from build123d import *

# Parameters (mm, degrees)
SKIZZE2_W                       = 28
SKIZZE2_H                       = 4
AUFSATZ_LINEAR_AUSTRAGEN2_DEPTH = 17.9
SKIZZE4_W                       = 35.8
SKIZZE4_H                       = 28
AUFSATZ_LINEAR_AUSTRAGEN3_DEPTH = 5
SKIZZE7_W                       = 8.2
SKIZZE7_H                       = 3
SCHNITT_LINEAR_AUSTRAGEN4_DEPTH = 1.5
SKIZZE5_W                       = 33.2
SKIZZE5_H                       = 18.5
SCHNITT_LINEAR_AUSTRAGEN2_DEPTH = 4.3
SKIZZE8_W                       = 34.6
SKIZZE8_H                       = 28
SCHNITT_LINEAR_AUSTRAGEN5_DEPTH = 3.5
AUFSATZ_LINEAR_AUSTRAGEN4_DEPTH = 1.5
SKIZZE9_W                       = 33.2
SKIZZE9_H                       = 3
SCHNITT_LINEAR_AUSTRAGEN6_DEPTH = 1.5
SKIZZE11_W                      = 28
SKIZZE11_H                      = 4.8
AUFSATZ_LINEAR_AUSTRAGEN5_DEPTH = 1.2
SKIZZE12_W                      = 28
SKIZZE12_H                      = 4.75
AUFSATZ_LINEAR_AUSTRAGEN6_DEPTH = 3.65
SKIZZE13_R                      = 1.2
AUFSATZ_LINEAR_AUSTRAGEN7_DEPTH = 2.5
LINEARES_MUSTER1_COUNT          = 2
LINEARES_MUSTER1_PITCH          = 15.2
LINEARES_MUSTER1_COUNT_DIR2     = 2
LINEARES_MUSTER1_PITCH_DIR2     = 21.6
SCHNITT_LINEAR_AUSTRAGEN7_DEPTH = 14.8
VERRUNDUNG1_R                   = 0.2
SKIZZE20_W                      = 27.6
SKIZZE20_H                      = 4.65
AUFSATZ_LINEAR_AUSTRAGEN8_DEPTH = 1.3
VERRUNDUNG2_R                   = 1.5
SCHNITT_LINEAR_AUSTRAGEN8_DEPTH = 1


with BuildPart() as part:
    # Skizze2 → Aufsatz-Linear austragen2 (new body, symmetric)
    with BuildSketch(Plane(origin=(0, 0, 0), x_dir=(0, 0, -1), z_dir=(1, 0, 0))):
        with Locations((0, -2)):
            Rectangle(SKIZZE2_W, SKIZZE2_H)
    extrude(amount=AUFSATZ_LINEAR_AUSTRAGEN2_DEPTH, both=True)

    # Skizze4 → Aufsatz-Linear austragen3 (add)
    with BuildSketch(Plane(origin=(0, 0, 0), x_dir=(1, 0, 0), z_dir=(0, 1, 0))):
        Rectangle(SKIZZE4_W, SKIZZE4_H)
    extrude(amount=AUFSATZ_LINEAR_AUSTRAGEN3_DEPTH)

    # Skizze7 → Schnitt-Linear austragen4 (cut)
    with BuildSketch(Plane.ZY.offset(17.9)):
        with Locations((0, 3.5)):
            Rectangle(SKIZZE7_W, SKIZZE7_H)
    extrude(amount=-SCHNITT_LINEAR_AUSTRAGEN4_DEPTH, mode=Mode.SUBTRACT)

    # Skizze5 → Schnitt-Linear austragen2 (cut)
    with BuildSketch(Plane(origin=(0, 5, 0), x_dir=(1, 0, 0), z_dir=(0, 1, 0))):
        with Locations((-0.1, 0)):
            Rectangle(SKIZZE5_W, SKIZZE5_H)
    extrude(amount=-SCHNITT_LINEAR_AUSTRAGEN2_DEPTH, mode=Mode.SUBTRACT)

    # Skizze8 → Schnitt-Linear austragen5 (cut)
    with BuildSketch(Plane(origin=(0, 5, 0), x_dir=(1, 0, 0), z_dir=(0, 1, 0))):
        with Locations((0.6, 0)):
            Rectangle(SKIZZE8_W, SKIZZE8_H)
    extrude(amount=-SCHNITT_LINEAR_AUSTRAGEN5_DEPTH, mode=Mode.SUBTRACT)

    # Skizze10 → Aufsatz-Linear austragen4 (add, symmetric)
    with BuildSketch(Plane.XY):
        Polygon((17.9, 1.5), (16.5, 1.5), (16.5, 2.5), (16.2, 2.5), (16.491176187, 3.3), (17.9, 3.3), align=None)
    extrude(amount=AUFSATZ_LINEAR_AUSTRAGEN4_DEPTH, both=True)

    # Skizze9 → Schnitt-Linear austragen6 (cut)
    with BuildSketch(Plane(origin=(0, 0.7, 0), x_dir=(1, 0, 0), z_dir=(0, 1, 0))):
        with Locations((-0.1, -7.75)):
            Rectangle(SKIZZE9_W, SKIZZE9_H)
        with Locations((-0.1, 7.75)):
            Rectangle(SKIZZE9_W, SKIZZE9_H)
    extrude(amount=-SCHNITT_LINEAR_AUSTRAGEN6_DEPTH, mode=Mode.SUBTRACT)

    # Skizze11 → Aufsatz-Linear austragen5 (add)
    with BuildSketch(Plane.ZY.offset(17.9)):
        with Locations((0, 7.4)):
            Rectangle(SKIZZE11_W, SKIZZE11_H)
    extrude(amount=-AUFSATZ_LINEAR_AUSTRAGEN5_DEPTH)

    # Skizze12 → Aufsatz-Linear austragen6 (add)
    with BuildSketch(Plane(origin=(0, 1.5, 0), x_dir=(1, 0, 0), z_dir=(0, 1, 0))):
        with Locations((-2.7, 11.625)):
            Rectangle(SKIZZE12_W, SKIZZE12_H)
        with Locations((-2.7, -11.625)):
            Rectangle(SKIZZE12_W, SKIZZE12_H)
    extrude(amount=AUFSATZ_LINEAR_AUSTRAGEN6_DEPTH)

    # Skizze13 → Aufsatz-Linear austragen7 (add)
    with BuildSketch(Plane(origin=(0, 5.15, 0), x_dir=(1, 0, 0), z_dir=(0, 1, 0))):
        with Locations((-6.5, 10.8)):
            Circle(SKIZZE13_R)
    aufsatz_linear_austragen7 = extrude(amount=AUFSATZ_LINEAR_AUSTRAGEN7_DEPTH)

    # Lineares Muster1: Aufsatz-Linear austragen7 2 × 2
    with Locations(*[(i * LINEARES_MUSTER1_PITCH, 0, j * LINEARES_MUSTER1_PITCH_DIR2) for i in range(LINEARES_MUSTER1_COUNT) for j in range(LINEARES_MUSTER1_COUNT_DIR2) if (i, j) != (0, 0)]):
        add(aufsatz_linear_austragen7)

    # Skizze14 → Schnitt-Linear austragen7 (cut, through all)
    with BuildSketch(Plane.XZ.offset(4)):
        Polygon((-17.9, -14), (-17.9, -13.8), (-14.51944695, -13.8), (-14.4, -13.95), (-13.4, -13.8), (9.48055305, -13.8), (9.6, -13.95), (10.6, -13.8), (17.9, -13.8), (17.9, -14), align=None)
        Polygon((10.6, 13.8), (17.9, 13.8), (17.9, 14), (-17.9, 14), (-17.9, 13.8), (-14.51944695, 13.8), (-14.4, 13.95), (-13.4, 13.8), (9.48055305, 13.8), (9.6, 13.95), align=None)
    extrude(amount=-SCHNITT_LINEAR_AUSTRAGEN7_DEPTH, mode=Mode.SUBTRACT)

    # Verrundung1
    verrundung1_edges = [part.edges().sort_by_distance(p)[0] for p in [
        (-14.4, 0.575, -13.95),
        (9.6, 0.575, -13.95),
        (9.6, 0.575, 13.95),
        (-14.4, 0.575, 13.95),
    ]]
    fillet(verrundung1_edges, radius=VERRUNDUNG1_R)

    # Skizze20 → Aufsatz-Linear austragen8 (add)
    with BuildSketch(Plane(origin=(-16.7, 0, 0), x_dir=(0, 0, -1), z_dir=(1, 0, 0))):
        with Locations((0, 7.475)):
            Rectangle(SKIZZE20_W, SKIZZE20_H)
    extrude(amount=AUFSATZ_LINEAR_AUSTRAGEN8_DEPTH)

    # Verrundung2
    verrundung2_edges = [part.edges().sort_by_distance(p)[0] for p in [
        (-16.65, 9.8, -13.8),
        (-16.65, 9.8, 13.8),
    ]]
    fillet(verrundung2_edges, radius=VERRUNDUNG2_R)

    # Skizze21 → Schnitt-Linear austragen8 (cut)
    with BuildSketch(Plane.ZY.offset(17.9)):
        Polygon((-13.218058581, -3.5), (-13.218058581, 0.095646159), (-12.710980277, 0.095646159), (-12.710980277, -3.085117751), (-11.005353253, -3.085117751), (-11.005353253, -3.5), align=None)
    extrude(amount=-SCHNITT_LINEAR_AUSTRAGEN8_DEPTH, mode=Mode.SUBTRACT)


solid = part.part
Verification items for the finished model (mm, model axes). A direction names the side the tool comes from. Give positions to 0.01 mm unless a question says otherwise; leave off trailing zeros. Loops run counter-clockwise (first coordinate to the right, second up) from the corner with the lowest first, then second, coordinate; pieces in that order, holes last.
1) Sectioned sample at B-B, the plane x = 4. Enter the section's corners in (y, z), then the cut area to 3 significant figures.
2) Depth check by flat-ended pin: pin 1 Ø0.5 at (x, y) = (-17, -3) entering from -Z; pin 2 Ø3.5 at (x, z) = (1, 10.5) entering from +Y; pin 3 Ø0.6 at (x, y) = (-17, 3.5) entering from +Z; pin 4 Ø3 at (x, y) = (-11, 7) entering from +Z. Enter the tip coordinate at first touch or a pass-through.
3) Sectioned sample at D-D, the plane z = -8. Enter the section's corners in (x, y), then the cut area to 3 significant figures.
4) Sectioned sample at A-A, the plane z = 3.25. Enter the section's corners in (x, y), then the cut area to 3 significant figures.
5) Draft check along Y on faces 1 (the flat face through (-17.4, -1.7, -13.218)), 2 (the flat face through (-17, 9.8, 0)), 3 (the cylindrical face through (8.44, 6.38, 11.97)). Enter one of: pulls with the +Y half, pulls with the -Y half, needs draft (parallel to the pull), parting line crosses it, or undercut.
6) Sectioned sample at C-C, the plane z = 10.8. Enter the section's corners in (x, y), then the cut area to 3 significant figures.
7) Set-up check for faces 4 (the flat face through (-16.7, 1.6, -0.1)), 5 (the flat face through (-17, 3, -4.1)), 6 (the flat face through (-13.849, 0.511, 13.867)), 7 (the flat face through (-16, 5.15, 0)), 8 (the flat face through (-17.4, -3.5, -12.1)): record each of +Z, -Z, +X, -X, +Y, -Y from which the full face is reachable in a straight line by a thin tool's end or side.
8) Thickness scan on line 1 along Z through (x, y) = (-9, -0.5); line 2 along Z through (x, y) = (11, 0.75); line 3 along X through (y, z) = (7.25, -11.25). Record the ranges inside material, lowest first.
Answers:
1. outline: (-4, -13.8) - (5.15, -13.8) - (5.15, -9.25) - (-0.8, -9.25) - (-0.8, -6.25) - (0.7, -6.25) - (0.7, 6.25) - (-0.8, 6.25) - (-0.8, 9.25) - (5.15, 9.25) - (5.15, 13.8) - (-4, 13.8) - close
1. area: 161 mm2
2. pin 1: stops at z = -13.8
2. pin 2: stops at y = 5.15
2. pin 3: stops at z = 13.8
2. pin 4: passes through
3. outline: (-17.9, -4) - (17.9, -4) - (17.9, 1.5) - (16.5, 1.5) - (16.5, -0.8) - (-16.7, -0.8) - (-16.7, 5.15) - (-15.4, 5.15) - (-15.4, 9.8) - (-17.9, 9.8) - close
3. area: 137 mm2
4. outline: (-17.9, -4) - (17.9, -4) - (17.9, 1.5) - (16.5, 1.5) - (16.5, 0.7) - (-16.7, 0.7) - (-16.7, 2) - (-17.9, 2) - close; (-17.9, 5) - (-16.7, 5) - (-16.7, 5.15) - (-15.4, 5.15) - (-15.4, 9.8) - (-17.9, 9.8) - close
4. area: 183 mm2
5. face 1: undercut
5. face 2: pulls with the +Y half
5. face 3: needs draft
6. outline: (-17.9, -4) - (17.9, -4) - (17.9, 1.5) - (11.3, 1.5) - (11.3, 5.15) - (9.9, 5.15) - (9.9, 7.65) - (7.5, 7.65) - (7.5, 5.15) - (-5.3, 5.15) - (-5.3, 7.65) - (-7.7, 7.65) - (-7.7, 5.15) - (-15.4, 5.15) - (-15.4, 9.8) - (-17.9, 9.8) - close
6. area: 327 mm2
7. face 4: none
7. face 5: +X, -X
7. face 6: +Z, +Y, -Y
7. face 7: +X
7. face 8: -X
8. line 1: z = -13.8 to -9.25, -6.25 to 6.25, 9.25 to 13.8
8. line 2: z = -13.8 to -9.25, 9.25 to 13.8
8. line 3: x = -17.9 to -15.4, -7.61 to -5.39, 7.59 to 9.81
